For this review, take the finished solid that the model builds, in its own axes (mm). Face numbers are marked on the shaded views. A direction names the side the tool comes from. Coordinates: 2 decimals unless noted, no trailing zeros. Write each loop counter-clockwise with the first axis right and the second up, starting at its lowest first coordinate (ties: lowest second). Pieces come first, ordered by that corner, then holes.
1) Mouldability with a two-part tool opening along Z and no side actions: class the marked faces 3, 4 and 5 as pulls with the +Z half, pulls with the -Z half, needs draft (parallel to the pull), parting line crosses it, or undercut.
2) To check wall thickness, follow line 1 along Z through (x, y) = (2, 2.5); line 2 along X through (y, z) = (-0.2, 0); line 3 along X through (y, z) = (12.5, -0.25). State the ranges of each line that lie inside material, in increasing order.
3) We need section D-D on x = 2. Write out the cut boundary in (y, z), then the cut area to 3 significant figures.
4) We need section B-B on y = 13. Write out the cut boundary in (x, z), then the cut area to 3 significant figures.
5) We need section C-C on x = 0. Write out the cut boundary in (y, z), then the cut area to 3 significant figures.
6) Insertion check: P1, Ø0.5, axis at x = 9.5, z = -1.5, coming from the +Y side; P2, Ø6, axis at x = -1, z = 0, coming from the +Y side. Each pin has a flat end and moves straight along its axis. Give the tip position at first contact, or say it passes through.
7) For the marked faces 1 and 2, list the 3-axis set-ups (+Z, -Z, +X, -X, +Y, -Y) from which the entire face can be reached by the end or side of a thin tool; tool diameter is ignored.
8) We need section A-A on z = 0. Write out the cut boundary in (x, y).
from build123d import *

# Parameters (mm, degrees)
BOSS_EXTRUDE1_DEPTH = 21
BOSS_EXTRUDE2_START = -0.3
SKETCH3_R           = 0.9
BOSS_EXTRUDE2_DEPTH = 0.3
CUT_EXTRUDE1_DEPTH  = 2


with BuildPart() as part:
    # Sketch2 → Boss-Extrude1 (new body)
    with BuildSketch(Plane(origin=(0, 0, 0), x_dir=(1, 0, 0), z_dir=(0, 1, 0))):
        with BuildLine():
            Line((-6.55, 7.3), (6.55, 7.3))
            ThreePointArc((6.55, 7.3), (9.75, 0), (6.55, -7.3))
            Line((6.55, -7.3), (-6.55, -7.3))
            ThreePointArc((-6.55, -7.3), (-9.75, 0), (-6.55, 7.3))
        make_face()
        with BuildLine():
            Line((-6.55, 7), (6.55, 7))
            ThreePointArc((6.55, 7), (9.449494937, 0), (6.55, -7))
            Line((6.55, -7), (-6.55, -7))
            ThreePointArc((-6.55, -7), (-9.449494937, 0), (-6.55, 7))
        make_face(mode=Mode.SUBTRACT)
    extrude(amount=BOSS_EXTRUDE1_DEPTH)

    # Sketch3 → Boss-Extrude2 (add)
    with BuildSketch(Plane(origin=(0, 0, 0), x_dir=(1, 0, 0), z_dir=(0, 1, 0)).offset(BOSS_EXTRUDE2_START)):
        with BuildLine():
            Line((-6.55, 7.3), (6.55, 7.3))
            ThreePointArc((6.55, 7.3), (9.75, 0), (6.55, -7.3))
            Line((6.55, -7.3), (-6.55, -7.3))
            ThreePointArc((-6.55, -7.3), (-9.75, 0), (-6.55, 7.3))
        make_face()
        with Locations(Location((0, 0, 0), (0, 0, 270))):
            Circle(SKETCH3_R, mode=Mode.SUBTRACT)
    extrude(amount=BOSS_EXTRUDE2_DEPTH)

    # Sketch4 → Cut-Extrude1 (cut)
    with BuildSketch(Plane(origin=(0, 21, 0), x_dir=(1, 0, 0), z_dir=(0, 1, 0))):
        Polygon((-7.631188375, 1), (-14.631115783, 1), (-14.631115783, -1), (-7.538875612, -1), (-7.538875612, -2), (-15.384565747, -2), (-15.384565747, 2), (-7.631188375, 2), align=None)
        Polygon((7.631188375, 2), (7.631188375, 1), (14.631115783, 1), (14.631115783, -1), (7.538875612, -1), (7.538875612, -2), (15.384565747, -2), (15.384565747, 2), align=None)
    extrude(amount=-CUT_EXTRUDE1_DEPTH, mode=Mode.SUBTRACT)


solid = part.part
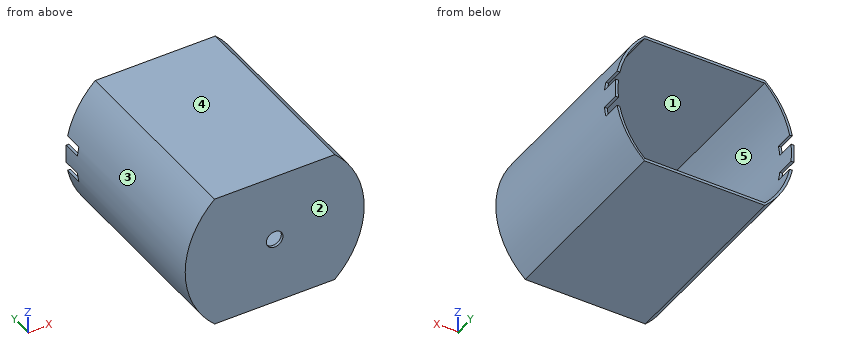
Result:
1. face 3: parting line crosses it
1. face 4: pulls with the +Z half
1. face 5: undercut
2. line 1: z = -7.3 to -7, 7 to 7.3
2. line 2: x = -9.75 to -0.9, 0.9 to 9.75
2. line 3: x = -9.75 to -9.45, 9.45 to 9.75
3. outline: (-0.3, -7.3) - (21, -7.3) - (21, -7) - (0, -7) - (0, 7) - (21, 7) - (21, 7.3) - (-0.3, 7.3) - close
3. area: 17.0 mm2
4. outline: (-6.55, -7.3) - (6.55, -7.3) arc R9.93 ccw to (6.55, 7.3) - (-6.55, 7.3) arc R9.93 ccw to start; hole (-6.55, -7) - (6.55, -7) arc R9.9 ccw to (6.55, 7) - (-6.55, 7) arc R9.9 ccw to start
4. area: 16.5 mm2
5. outline: (-0.3, -7.3) - (21, -7.3) - (21, -7) - (0, -7) - (0, -0.9) - (-0.3, -0.9) - close; (-0.3, 0.9) - (0, 0.9) - (0, 7) - (21, 7) - (21, 7.3) - (-0.3, 7.3) - close
5. area: 16.4 mm2
6. P1: stops at y = 19
6. P2: stops at y = 0
7. face 1: +Y
7. face 2: +Z, -Z, +X, -X, -Y
8. outline: (-9.75, -0.3) - (-0.9, -0.3) - (-0.9, 0) - (-9.45, 0) - (-9.45, 21) - (-9.75, 21) - close; (0.9, -0.3) - (9.75, -0.3) - (9.75, 21) - (9.45, 21) - (9.45, 0) - (0.9, 0) - close
